Input: part model. Units: mm. Frame: model coordinates. A direction names the side the tool comes from. Round coordinates to 2 decimals unless told otherwise and drop trailing zeros. Write each loop counter-clockwise with the first axis right and the second up, starting at its lowest first coordinate (ties: lowest second). Pieces come first, ordered by that corner, then holes. Notation, with made-up numbers: (32, -37.5) -> (57, -37.5) arc R24 ccw to (57, -6.5) -> close; hole circle Ø10 at (-28, -1). An arc over 180 degrees is marked (long way). Write item = value, one per line. Start each with the question number.
```python
from build123d import *

# Parameters (mm, degrees)
SKETCH1_R           = 14
BOSS_EXTRUDE1_DEPTH = 5
SKETCH2_R           = 9.6
BOSS_EXTRUDE2_DEPTH = 0.5
SKETCH3_R           = 8.475
BOSS_EXTRUDE3_DEPTH = 5
SKETCH4_R           = 1.4
CUT_EXTRUDE1_DEPTH  = 21.548722588
CIRPATTERN1_COUNT   = 4
SKETCH5_R           = 2.5
CUT_EXTRUDE2_DEPTH  = 21.548722588
CHAMFER1_SIZE       = 0.6
SKETCH6_R           = 4.25
CUT_EXTRUDE3_DEPTH  = 2.5
SKETCH7_R           = 2.3
CUT_EXTRUDE4_DEPTH  = 6.5
SKETCH8_R           = 1.5
SKETCH8_R_2         = 1.2
BOSS_EXTRUDE4_DEPTH = 3.5


with BuildPart() as part:
    # Sketch1 → Boss-Extrude1 (new body)
    with BuildSketch(Plane(origin=(0, 0, 0), x_dir=(1, 0, 0), z_dir=(0, 1, 0))):
        with Locations(Location((0, 0, 0), (0, 0, 270))):
            Circle(SKETCH1_R)
    extrude(amount=BOSS_EXTRUDE1_DEPTH)

    # Sketch2 → Boss-Extrude2 (add)
    with BuildSketch(Plane(origin=(0, 5, 0), x_dir=(1, 0, 0), z_dir=(0, 1, 0))):
        with Locations(Location((1.5, 0, 0), (0, 0, 270))):
            Circle(SKETCH2_R)
    extrude(amount=BOSS_EXTRUDE2_DEPTH)

    # Sketch3 → Boss-Extrude3 (add)
    with BuildSketch(Plane(origin=(0, 5.5, 0), x_dir=(1, 0, 0), z_dir=(0, 1, 0))):
        with Locations(Location((1.5, 0, 0), (0, 0, 270))):
            Circle(SKETCH3_R)
    extrude(amount=BOSS_EXTRUDE3_DEPTH)

    # Sketch4 → Cut-Extrude1 (cut, through all)
    with BuildSketch(Plane(origin=(0, 5, 0), x_dir=(1, 0, 0), z_dir=(0, 1, 0))):
        with Locations(Location((-7.071067812, 7.071067812, 0), (0, 0, 270))):
            Circle(SKETCH4_R)
    cut_extrude1 = extrude(amount=-CUT_EXTRUDE1_DEPTH, mode=Mode.SUBTRACT)

    # CirPattern1: Cut-Extrude1 ×4 about axis
    cirpattern1_axis = Axis((0, 0, 0), (0, 1, 0))
    for i in range(1, CIRPATTERN1_COUNT):
        add(cut_extrude1.rotate(cirpattern1_axis, i * 360 / CIRPATTERN1_COUNT), mode=Mode.SUBTRACT)

    # Sketch5 → Cut-Extrude2 (cut, through all)
    with BuildSketch(Plane(origin=(0, 5, 0), x_dir=(1, 0, 0), z_dir=(0, 1, 0))):
        with Locations((-7.071067812, 7.071067812)):
            Circle(SKETCH5_R)
        with Locations((7.071067812, 7.071067812)):
            Circle(SKETCH5_R)
        with Locations((7.071067812, -7.071067812)):
            Circle(SKETCH5_R)
        with Locations((-7.071067812, -7.071067812)):
            Circle(SKETCH5_R)
    extrude(amount=CUT_EXTRUDE2_DEPTH, mode=Mode.SUBTRACT)

    # Chamfer1
    chamfer1_edges = [part.edges().sort_by_distance(p)[0] for p in [
        (-7.071067812, 5, -8.471067812),
        (8.471067812, 5, -7.071067812),
        (7.071067812, 5, 8.471067812),
        (-8.471067812, 5, 7.071067812),
    ]]
    chamfer(chamfer1_edges, length=CHAMFER1_SIZE)

    # Sketch6 → Cut-Extrude3 (cut)
    with BuildSketch(Plane.XZ):
        with Locations(Location((0, 0, 0), (0, 0, 270))):
            Circle(SKETCH6_R)
    extrude(amount=-CUT_EXTRUDE3_DEPTH, mode=Mode.SUBTRACT)

    # Sketch7 → Cut-Extrude4 (cut)
    with BuildSketch(Plane(origin=(0, 10.5, 0), x_dir=(1, 0, 0), z_dir=(0, 1, 0))):
        with Locations(Location((0, 0, 0), (0, 0, 270))):
            Circle(SKETCH7_R)
    extrude(amount=-CUT_EXTRUDE4_DEPTH, mode=Mode.SUBTRACT)

    # Sketch8 → Boss-Extrude4 (add)
    with BuildSketch(Plane(origin=(0, 10.5, 0), x_dir=(1, 0, 0), z_dir=(0, 1, 0))):
        with Locations(Location((0, 5.8, 0), (0, 0, 270))):
            Circle(SKETCH8_R)
        with Locations(Location((0, -5.8, 0), (0, 0, 270))):
            Circle(SKETCH8_R_2)
    extrude(amount=BOSS_EXTRUDE4_DEPTH)


solid = part.part
```
1. Section D-D (x = 0). Output: boundary loops of the cut face in (y, z), then the cut area to 3 significant figures.
2. Reachability of faces 5 (the cylindrical face through (0.45, 12.23, -4.37)), 6 (the cylindrical face through (0.076, 5.246, 9.494)), 7 (the cylindrical face through (-6.32, 2.23, 5.89)), 8 (the flat face through (0, 2.5, 0)) from +Z, -Z, +X, -X, +Y, -Y: full face, straight path, thin tool, end or side. Return the list, or none.
3. Section A-A (z = 0). Output: boundary loops of the cut face in (x, y) (3 decimals), then the cut area to 3 significant figures.
4. Section B-B (y = 13). Output: boundary loops of the cut face in (x, z).
5. Mould query, pull axis Z, two halves, no side actions, for faces 1 (the cylindrical face through (9.975, 7.965, 0.074)), 2 (the cylindrical face through (0.221, 5.246, -9.514)), 3 (the cylindrical face through (5.478, 7.712, -5.144)), 4 (the flat face through (10.4, 5.5, -0.1)). Classes: pulls with the +Z half, pulls with the -Z half, needs draft (parallel to the pull), parting line crosses it, or undercut.
6. Pin query (flat end, axial travel): P1, Ø3.5, axis at x = -1, z = 0, coming from the +Y side; P2, Ø4.5, axis at x = 7.07, z = 7.07, coming from the +Y side; P3, Ø6, axis at y = 6, z = 5.5, coming from the +X side; P4, Ø10, axis at x = 0, z = 0, coming from the +Y side. Return the tip coordinate at first contact, or that it passes through.
7. Line query: line 1 along Y through (x, z) = (-11, -3.25); line 2 along Z through (x, y) = (1, 12.75); line 3 along X through (y, z) = (8.25, 0) (3 decimals). Output: solid intervals per line, ascending.
Check sheet entries:
q1.outline = (0, -14) -> (5, -14) -> (5, -9.48) -> (5.5, -9.48) -> (5.5, -8.34) -> (10.5, -8.34) -> (10.5, -7.3) -> (14, -7.3) -> (14, -4.3) -> (10.5, -4.3) -> (10.5, -2.3) -> (4, -2.3) -> (4, 2.3) -> (10.5, 2.3) -> (10.5, 4.6) -> (14, 4.6) -> (14, 7) -> (10.5, 7) -> (10.5, 8.34) -> (5.5, 8.34) -> (5.5, 9.48) -> (5, 9.48) -> (5, 14) -> (0, 14) -> (0, 4.25) -> (2.5, 4.25) -> (2.5, -4.25) -> (0, -4.25) -> close
q1.area = 201 mm2
q2.face_5 = +Y
q2.face_6 = +Z, +Y
q2.face_7 = +Y, -Y
q2.face_8 = -Y
q3.outline = (-14, 0) -> (-4.25, 0) -> (-4.25, 2.5) -> (4.25, 2.5) -> (4.25, 0) -> (14, 0) -> (14, 5) -> (11.1, 5) -> (11.1, 5.5) -> (9.975, 5.5) -> (9.975, 10.5) -> (2.3, 10.5) -> (2.3, 4) -> (-2.3, 4) -> (-2.3, 10.5) -> (-6.975, 10.5) -> (-6.975, 5.5) -> (-8.1, 5.5) -> (-8.1, 5) -> (-14, 5) -> close
q3.area = 183 mm2
q4.outline = circle Ø3 at (0, -5.8); circle Ø2.4 at (0, 5.8)
q5.face_1 = parting line crosses it
q5.face_2 = pulls with the -Z half
q5.face_3 = undercut
q5.face_4 = needs draft
q6.P1 = 10.5
q6.P2 = 5
q6.P3 = 13.74
q6.P4 = 14
q7.line_1 = 0 to 5
q7.line_2 = -6.92 to -4.68, 5.14 to 6.46
q7.line_3 = -6.975 to -2.3, 2.3 to 9.975
